```python
from build123d import *

# Parameters (mm, degrees)
SKETCH1_R             = 20.5
SKETCH1_R_2           = 17.5
BOSS_EXTRUDE1_DEPTH   = 9
SKETCH1_R_3           = 28.5
SKETCH1_R_4           = 25.5
BOSS_EXTRUDE1_2_DEPTH = 9
BOSS_EXTRUDE2_START   = 0.5
SKETCH1_3_R           = 25.5
SKETCH1_3_R_2         = 20.5
BOSS_EXTRUDE2_DEPTH   = 8


with BuildPart() as part:
    # Sketch1 → Boss-Extrude1 (new body)
    with BuildSketch(Plane(origin=(0, 0, 0), x_dir=(0, 1, 0), z_dir=(0, 0, 1))):
        Circle(SKETCH1_R)
        Circle(SKETCH1_R_2, mode=Mode.SUBTRACT)
    extrude(amount=BOSS_EXTRUDE1_DEPTH)



with BuildPart() as body_2:
    # Sketch1 → Boss-Extrude1 2 (new body)
    with BuildSketch(Plane(origin=(0, 0, 0), x_dir=(0, 1, 0), z_dir=(0, 0, 1))):
        Circle(SKETCH1_R_3)
        Circle(SKETCH1_R_4, mode=Mode.SUBTRACT)
    extrude(amount=BOSS_EXTRUDE1_2_DEPTH)


with BuildPart() as part_1:
    add(part.part)

    add(body_2.part)  # Boss-Extrude2 merges body 2
    # Sketch1_3 → Boss-Extrude2 (add)
    with BuildSketch(Plane(origin=(0, 0, 0), x_dir=(0, 1, 0), z_dir=(0, 0, 1)).offset(BOSS_EXTRUDE2_START)):
        Circle(SKETCH1_3_R)
        Circle(SKETCH1_3_R_2, mode=Mode.SUBTRACT)
    extrude(amount=BOSS_EXTRUDE2_DEPTH)


solid = part_1.part
```
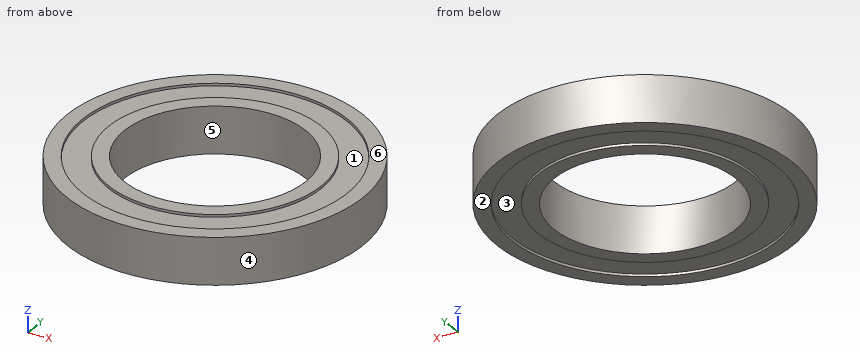
Could you check a few things on this model? Use its own coordinates, in mm. Face numbers are marked on the shaded views. A direction names the side the tool comes from. Round coordinates to 2 decimals unless told otherwise and drop trailing zeros. Loops run counter-clockwise (first coordinate to the right, second up) from the corner with the lowest first, then second, coordinate; pieces in that order, holes last.
Q1. I want a section at D-D (x = -19). Write out the boundary of the cut face in (y, z).
Q2. Thinking about a two-plate mould opening in Y: for the marked faces 4, 5 and 6, which applies, pulls with the +Y half, pulls with the -Y half, needs draft (parallel to the pull), parting line crosses it, or undercut?
Q3. Please list where these lines run through material, in increasing order: L1, parallel to Y at x = 0, z = 8.6; L2, parallel to Y at x = 0, z = 5.25.
Q4. I want a section at C-C (z = 1.75). Write out the boundary of the cut face in (x, y).
Q5. On a 3-axis mill with a long thin cutter (end or side, diameter ignored), from which of +Z, -Z, +X, -X, +Y, -Y can I reach the whole of each face in a straight line? I mean the marked faces 1, 2 and 3. Say none if no direction works.
Q6. I want a section at A-A (x = 0). Write out the boundary of the cut face in (y, z).
Q7. For P1, Ø15.5, axis at x = 5, y = 8, coming from the -Z side; P2, Ø5, axis at y = 11, z = 3.5, coming from the -X side; P3, Ø1.5, axis at y = -11.5, z = 4.5, coming from the -X side; P4, Ø2, axis at y = 4.5, z = 6.5, coming from the +X side, each with a flat end and sliding along its axis, tell me the tip position at first contact or that it passes through.
Answer below:
1. outline: (-21.24, 0) - (-17.01, 0) - (-17.01, 0.5) - (-7.7, 0.5) - (-7.7, 0) - (7.7, 0) - (7.7, 0.5) - (17.01, 0.5) - (17.01, 0) - (21.24, 0) - (21.24, 9) - (17.01, 9) - (17.01, 8.5) - (7.7, 8.5) - (7.7, 9) - (-7.7, 9) - (-7.7, 8.5) - (-17.01, 8.5) - (-17.01, 9) - (-21.24, 9) - close
2. face 4: parting line crosses it
2. face 5: undercut
2. face 6: needs draft
3. L1: y = -28.5 to -25.5, -20.5 to -17.5, 17.5 to 20.5, 25.5 to 28.5
3. L2: y = -28.5 to -17.5, 17.5 to 28.5
4. outline: circle Ø57 at (0, 0); hole circle Ø35 at (0, 0)
5. face 1: +Z
5. face 2: -Z, +X, -X, +Y, -Y
5. face 3: -Z
6. outline: (-28.5, 0) - (-25.5, 0) - (-25.5, 0.5) - (-20.5, 0.5) - (-20.5, 0) - (-17.5, 0) - (-17.5, 9) - (-20.5, 9) - (-20.5, 8.5) - (-25.5, 8.5) - (-25.5, 9) - (-28.5, 9) - close; (17.5, 0) - (20.5, 0) - (20.5, 0.5) - (25.5, 0.5) - (25.5, 0) - (28.5, 0) - (28.5, 9) - (25.5, 9) - (25.5, 8.5) - (20.5, 8.5) - (20.5, 9) - (17.5, 9) - close
7. P1: passes through
7. P2: stops at x = -27.2
7. P3: stops at x = -26.39
7. P4: stops at x = 28.28
